Check sheet for the drawn part. Datum: minimum x, y, z corner. Units: mm. Coordinates: 2 decimals unless noted, no trailing zeros. Loops run counter-clockwise (first coordinate to the right, second up) from the corner with the lowest first, then second, coordinate; pieces in that order, holes last. Notation, with made-up numbers: M 39,37.25 L 46,37.25 A17 cw 46,46.25 Z; hole C 45.5,64.25 d3. An arc over 180 degrees is marked long. Answer in a Markdown table with one row per item. Add a question column.
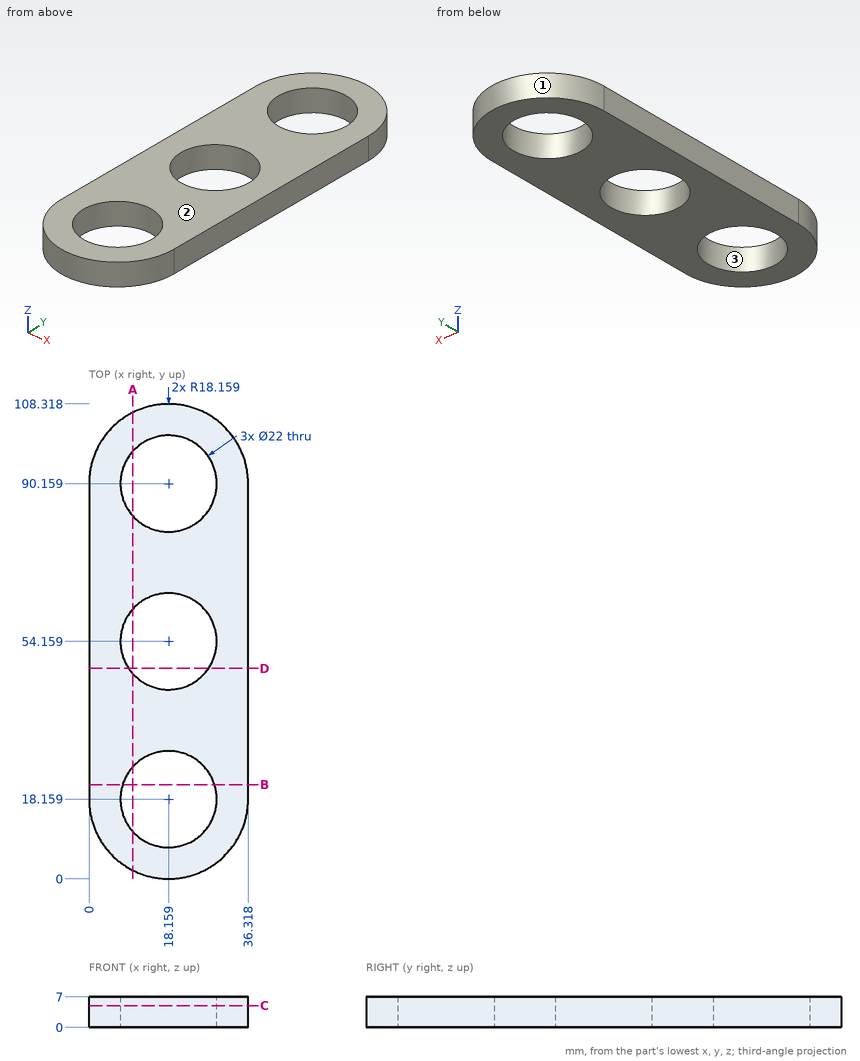
Q1. Cross-section at B-B (y = 21.5). Record the cut outline in (x, z), plus the area to 4 significant figures.
Q2. Thickness scan on L1, parallel to Y at x = 11, z = 0.5; L2, parallel to Y at x = 23.5, z = 5.5 (1 decimal); L3, parallel to X at y = 17.5, z = 4.5. Record the ranges inside material, lowest first.
Q3. Cross-section at D-D (y = 48). Record the cut outline in (x, z) (3 decimals).
Q4. Cross-section at A-A (x = 10). Record the cut outline in (y, z), plus the area to 3 significant figures.
Q5. Cross-section at C-C (z = 5). Record the cut outline in (x, y).
Q6. Mould release check, pull along Y, two halves, no side actions. Record for the marked faces 1, 2 and 3: released by +Y, released by -Y, zero draft, split by the parting line, or undercut.
Q7. Go/stop test with flat-tipped pins: pin 1 (1.5 mm diameter, centred on x = 16, z = 2.5, fed in from -Y); pin 2 (6 mm diameter, centred on x = 23, y = 86.5, fed in from -Z); pin 3 (1.5 mm diameter, centred on x = 11, z = 3, fed in from +Y). Record where each tip stops, or that it passes through.
Answer key:
| question | item | result |
|---|---|---|
| 1 | outline | M 0,0 L 7.68,0 L 7.68,7 L 0,7 Z; M 28.64,0 L 36.32,0 L 36.32,7 L 28.64,7 Z |
| 1 | area | 107.5 mm^2 |
| 2 | L1 | 1.47 to 9.81, 26.51 to 45.81, 62.51 to 81.81, 98.51 to 106.85 |
| 2 | L2 | 0.8 to 8.5, 27.8 to 44.5, 63.8 to 80.5, 99.8 to 107.5 |
| 2 | L3 | 0.01 to 7.18, 29.14 to 36.31 |
| 3 | outline | M 0,0 L 9.045,0 L 9.045,7 L 0,7 Z; M 27.273,0 L 36.318,0 L 36.318,7 L 27.273,7 Z |
| 4 | outline | M 1.94,0 L 10.78,0 L 10.78,7 L 1.94,7 Z; M 25.54,0 L 46.78,0 L 46.78,7 L 25.54,7 Z; M 61.54,0 L 82.78,0 L 82.78,7 L 61.54,7 Z; M 97.54,0 L 106.38,0 L 106.38,7 L 97.54,7 Z |
| 4 | area | 421 mm^2 |
| 5 | outline | M 0,18.16 A18.16 ccw 36.32,18.16 L 36.32,90.16 A18.16 ccw 0,90.16 Z; hole C 18.16,18.16 d22; hole C 18.16,54.16 d22; hole C 18.16,90.16 d22 |
| 6 | face 1 | released by +Y |
| 6 | face 2 | zero draft |
| 6 | face 3 | undercut |
| 7 | pin 1 | y = 0.05 |
| 7 | pin 2 | through |
| 7 | pin 3 | y = 107.15 |
